Input: dimensioned drawing with shaded views. Units: mm. Origin: part minimum x, y, z. Round coordinates to 2 decimals unless told otherwise and drop trailing zeros. Loops run counter-clockwise (first coordinate to the right, second up) from the corner with the lowest first, then second, coordinate; pieces in that order, holes last. Notation, with made-up numbers: M 65,82 L 76,82 A19 cw 76,113 Z; hole C -10.5,-9.5 d7. An arc over 180 degrees is marked long. Answer as a JSON object with one key per item and string values.
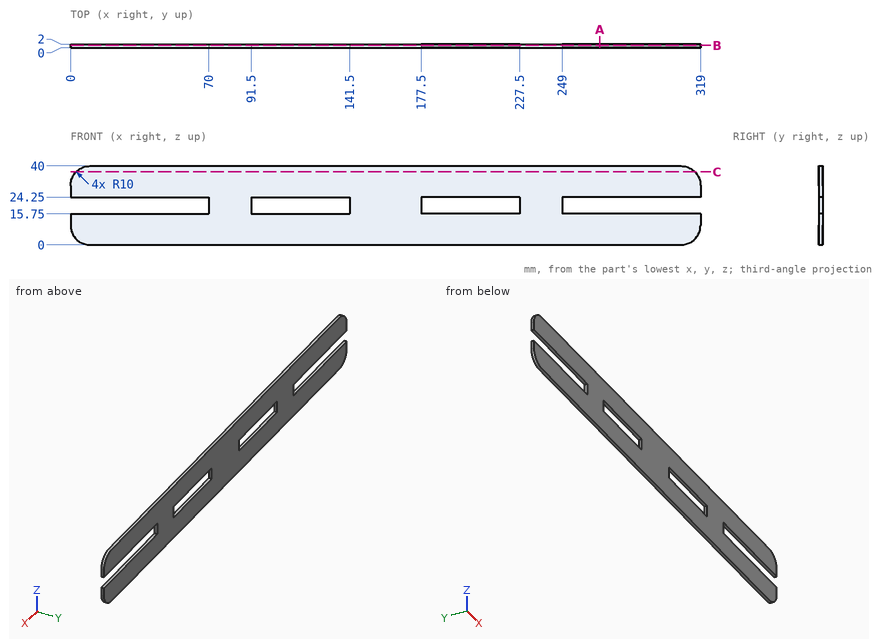
Item 1: Section C-C on z = 37. Return the cut outline in (x, y).
Answer sheet:
{"outline": "M 2.86,0 L 316.14,0 L 316.14,2 L 2.86,2 Z"}
Item 2: Section A-A on x = 268. Return the cut outline in (y, z), then the cut area to 3 significant figures.
Answer sheet:
{"outline": "M 0,0 L 2,0 L 2,15.75 L 0,15.75 Z; M 0,24.25 L 2,24.25 L 2,40 L 0,40 Z", "area": "63.0 mm²"}
Item 3: Contact query for flat-ended pins moving along their axis: pin 1 Ø0.6 at (y, z) = (0.5, 19) entering from +X; pin 2 Ø1 at (y, z) = (0.5, 18.5) entering from -X. Output: stop coordinate, or through.
Answer sheet:
{"pin 1": "stops at x = 249", "pin 2": "stops at x = 70"}
Item 4: Line query: probe 1 along X at (y, z) = (0.8, 23); probe 2 along Z at (x, y) = (281, 0.2); probe 3 along X at (y, z) = (1.2, 35). Output: solid intervals per line, ascending. Write a range as from..to.
Answer sheet:
{"probe 1": "x = 70..91.5, 141.5..177.5, 227.5..249", "probe 2": "z = 0..15.75, 24.25..40", "probe 3": "x = 1.34..317.66"}
Item 5: Section B-B on y = 1.25. Return the cut outline in (x, z), then the cut area to 3 significant figures.
Answer sheet:
{"outline": "M 0,10 A10 ccw 10,0 L 309,0 A10 ccw 319,10 L 319,15.75 L 249,15.75 L 249,24.25 L 319,24.25 L 319,30 A10 ccw 309,40 L 10,40 A10 ccw 0,30 L 0,24.25 L 70,24.25 L 70,15.75 L 0,15.75 Z; hole M 91.5,15.75 L 141.5,15.75 L 141.5,24.25 L 91.5,24.25 Z; hole M 177.5,15.75 L 227.5,15.75 L 227.5,24.25 L 177.5,24.25 Z", "area": "10,600 mm²"}
